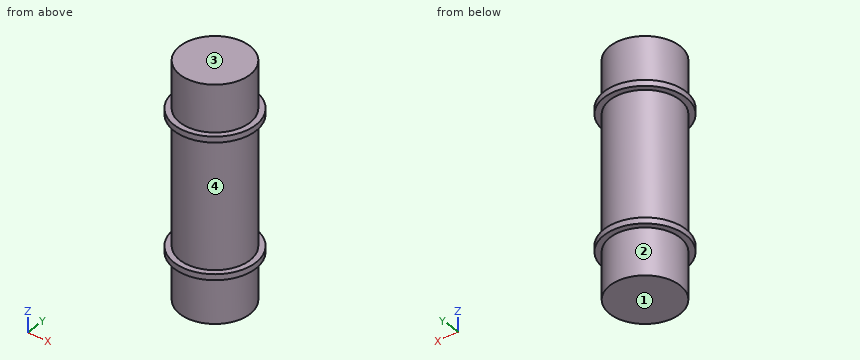
from build123d import *

# Parameters (mm, degrees)
ESQUISSE1_R        = 6
BOSS_EXTRU_1_DEPTH = 40
ESQUISSE2_R        = 7
ESQUISSE2_R_2      = 6
BOSS_EXTRU_2_DEPTH = 1
BOSS_EXTRU_3_START = -1
ESQUISSE3_R        = 7
ESQUISSE3_R_2      = 6
BOSS_EXTRU_3_DEPTH = 1


with BuildPart() as part:
    # Esquisse1 → Boss.-Extru.1 (new body)
    with BuildSketch(Plane.XY):
        Circle(ESQUISSE1_R)
    extrude(amount=BOSS_EXTRU_1_DEPTH)

    # Esquisse2 → Boss.-Extru.2 (add)
    with BuildSketch(Plane(origin=(0, 0, 8), x_dir=(-1, 0, 0), z_dir=(0, 0, -1))):
        Circle(ESQUISSE2_R)
        Circle(ESQUISSE2_R_2, mode=Mode.SUBTRACT)
    extrude(amount=-BOSS_EXTRU_2_DEPTH)

    # Esquisse3 → Boss.-Extru.3 (add)
    with BuildSketch(Plane.XY.offset(32).offset(BOSS_EXTRU_3_START)):
        with Locations(Location((0, 0, 0), (0, 0, 180))):
            Circle(ESQUISSE3_R)
        with Locations(Location((0, 0, 0), (0, 0, 180))):
            Circle(ESQUISSE3_R_2, mode=Mode.SUBTRACT)
    extrude(amount=BOSS_EXTRU_3_DEPTH)


solid = part.part
The listing builds one solid part. Answer for the finished solid, in the listing's coordinates (mm). Face numbers are marked on the shaded views. Coordinates: 2 decimals unless noted, no trailing zeros. Write each loop counter-clockwise with the first axis right and the second up, starting at its lowest first coordinate (ties: lowest second). Pieces come first, ordered by that corner, then holes. Notation, with made-up numbers: (-32, 43) - (1, 43) arc R17 cw to (1, 47) - close; hole circle Ø10 at (-13, 20). An arc over 180 degrees is marked (long way). Return JSON: item names as keys, results as strings.
1. The part is cut by section A-A on x = 0. Determine the outline of the cut face in (y, z), then the cut area to 3 significant figures.
Final values:
{"outline": "(-7, 8) - (-6, 8) - (-6, 0) - (6, 0) - (6, 8) - (7, 8) - (7, 9) - (6, 9) - (6, 31) - (7, 31) - (7, 32) - (6, 32) - (6, 40) - (-6, 40) - (-6, 32) - (-7, 32) - (-7, 31) - (-6, 31) - (-6, 9) - (-7, 9) - close", "area": "484 mm^2"}
2. Consider line 1 along Z through (x, y) = (6.5, 0.75); line 2 along Y through (x, z) = (2.25, 9.5); line 3 along X through (y, z) = (-1, 13). Determine where each line is inside the solid, lowest interval first.
Final values:
{"line 1": "8 to 9, 31 to 32", "line 2": "-5.56 to 5.56", "line 3": "-5.92 to 5.92"}
3. For a pull along Z with two mould halves and no side action, classify the marked faces 1, 2, 3 and 4 as +Z half, -Z half, draft (parallel to the pull), parting line (faces both ways), or undercut.
Final values:
{"face 1": "-Z half", "face 2": "draft", "face 3": "+Z half", "face 4": "undercut"}
4. Each of these flat-tipped pins is pushed along its axis until it touches: pin 1 Ø8 at (y, z) = (-3.5, 25.5) entering from -X; pin 2 Ø3 at (x, z) = (1.5, 19) entering from +Y; pin 3 Ø6 at (x, z) = (5, 10) entering from +Y. Where does it stop, or does it pass through?
Final values:
{"pin 1": "x = -6", "pin 2": "y = 6", "pin 3": "y = 6.65"}
5. The part is cut by section C-C on z = 6. Determine the outline of the cut face in (x, y).
Final values:
{"outline": "circle Ø12 at (0, 0)"}
